```python
from build123d import *

# Parameters (mm, degrees)
SKIZZE1_W                       = 10
SKIZZE1_H                       = 11
AUFSATZ_LINEAR_AUSTRAGEN1_DEPTH = 9
SKIZZE2_W                       = 1.5
SKIZZE2_H                       = 1
AUFSATZ_LINEAR_AUSTRAGEN2_DEPTH = 9
SKIZZE6_W                       = 3.75
SKIZZE6_H                       = 3.75
SCHNITT_LINEAR_AUSTRAGEN2_DEPTH = 10
LINEARES_MUSTER1_COUNT          = 4
LINEARES_MUSTER1_PITCH          = 4.25
LINEARES_MUSTER1_COUNT_DIR2     = 2
LINEARES_MUSTER1_PITCH_DIR2     = 4.25
SKIZZE7_W                       = 3.5
SKIZZE7_H                       = 3.5
AUFSATZ_LINEAR_AUSTRAGEN5_DEPTH = 9
LINEARES_MUSTER2_COUNT          = 3
LINEARES_MUSTER2_PITCH          = 4.25
LINEARES_MUSTER2_COUNT_DIR2     = 2
LINEARES_MUSTER2_PITCH_DIR2     = 4.25
AUFSATZ_LINEAR_AUSTRAGEN7_DEPTH = 9
LINEARES_MUSTER4_COUNT          = 4
LINEARES_MUSTER4_PITCH          = 4.25
LINEARES_MUSTER4_COUNT_DIR2     = 2
LINEARES_MUSTER4_PITCH_DIR2     = 4.25
SCHNITT_LINEAR_AUSTRAGEN4_DEPTH = 23.874658467
LINEARES_MUSTER6_COUNT          = 4
LINEARES_MUSTER6_PITCH          = 4.25
LINEARES_MUSTER6_COUNT_DIR2     = 2
LINEARES_MUSTER6_PITCH_DIR2     = 4.25
SKETCH_3_W                      = 20.071123044
SKETCH_3_H                      = 21.030403289
CUT_EXTRUDE_1_DEPTH             = 8


with BuildPart() as part:
    # Skizze1 → Aufsatz-Linear austragen1 (new, symmetric)
    with BuildSketch(Plane(origin=(0, 0, 0), x_dir=(0, 0, -1), z_dir=(1, 0, 0))):
        with Locations((0, 5.5)):
            Rectangle(SKIZZE1_W, SKIZZE1_H)
    extrude(amount=AUFSATZ_LINEAR_AUSTRAGEN1_DEPTH, both=True)

    # Skizze2 → Aufsatz-Linear austragen2 (add, symmetric)
    with BuildSketch(Plane(origin=(0, 0, 0), x_dir=(0, 0, -1), z_dir=(1, 0, 0))):
        with Locations((-5.75, 0.5)):
            Rectangle(SKIZZE2_W, SKIZZE2_H)
        with Locations((5.75, 0.5)):
            Rectangle(SKIZZE2_W, SKIZZE2_H)
    extrude(amount=AUFSATZ_LINEAR_AUSTRAGEN2_DEPTH, both=True)

    # Skizze6 → Schnitt-Linear austragen2 (cut)
    with BuildSketch(Plane.XZ):
        with Locations((-6.375, -2.125)):
            Rectangle(SKIZZE6_W, SKIZZE6_H)
    schnitt_linear_austragen2 = extrude(amount=-SCHNITT_LINEAR_AUSTRAGEN2_DEPTH, mode=Mode.SUBTRACT)

    # Lineares Muster1: Schnitt-Linear austragen2 4 × 2
    with Locations(*[(i * LINEARES_MUSTER1_PITCH, 0, j * LINEARES_MUSTER1_PITCH_DIR2) for i in range(LINEARES_MUSTER1_COUNT) for j in range(LINEARES_MUSTER1_COUNT_DIR2) if (i, j) != (0, 0)]):
        add(schnitt_linear_austragen2, mode=Mode.SUBTRACT)

    # Skizze7 → Aufsatz-Linear austragen5 (add)
    with BuildSketch(Plane(origin=(0, 11, 0), x_dir=(1, 0, 0), z_dir=(0, 1, 0))):
        with Locations((-6.375, -2.125)):
            Rectangle(SKIZZE7_W, SKIZZE7_H)
    aufsatz_linear_austragen5 = extrude(amount=AUFSATZ_LINEAR_AUSTRAGEN5_DEPTH)

    # Lineares Muster2: Aufsatz-Linear austragen5 3 × 2, 4 skipped
    with Locations(*[(i * LINEARES_MUSTER2_PITCH, 0, -j * LINEARES_MUSTER2_PITCH_DIR2) for i in range(LINEARES_MUSTER2_COUNT) for j in range(LINEARES_MUSTER2_COUNT_DIR2) if (i, j) not in ((0, 0), (0, 1), (1, 0), (1, 1), (2, 0))]):
        add(aufsatz_linear_austragen5)

    # Skizze10 → Aufsatz-Linear austragen7 (add)
    with BuildSketch(Plane(origin=(0, 11, 0), x_dir=(1, 0, 0), z_dir=(0, 1, 0))):
        Polygon((-4.625, 1.375), (-5.625, 0.375), (-7.125, 0.375), (-8.125, 1.375), (-8.125, 3.875), (-4.625, 3.875), align=None)
    aufsatz_linear_austragen7 = extrude(amount=AUFSATZ_LINEAR_AUSTRAGEN7_DEPTH)

    # Lineares Muster4: Aufsatz-Linear austragen7 4 × 2, 2 skipped
    with Locations(*[(i * LINEARES_MUSTER4_PITCH, 0, j * LINEARES_MUSTER4_PITCH_DIR2) for i in range(LINEARES_MUSTER4_COUNT) for j in range(LINEARES_MUSTER4_COUNT_DIR2) if (i, j) not in ((0, 0), (0, 1), (2, 0))]):
        add(aufsatz_linear_austragen7)

    # Skizze12 → Schnitt-Linear austragen4 (cut, through all)
    with BuildSketch(Plane(origin=(0, 20, 0), x_dir=(1, 0, 0), z_dir=(0, 1, 0))):
        Polygon((-5.875, 0.875), (-5.125, 1.625), (-5.125, 3.375), (-7.625, 3.375), (-7.625, 1.625), (-6.875, 0.875), align=None)
    schnitt_linear_austragen4 = extrude(amount=-SCHNITT_LINEAR_AUSTRAGEN4_DEPTH, mode=Mode.SUBTRACT)

    # Lineares Muster6: Schnitt-Linear austragen4 4 × 2
    with Locations(*[(i * LINEARES_MUSTER6_PITCH, 0, j * LINEARES_MUSTER6_PITCH_DIR2) for i in range(LINEARES_MUSTER6_COUNT) for j in range(LINEARES_MUSTER6_COUNT_DIR2) if (i, j) != (0, 0)]):
        add(schnitt_linear_austragen4, mode=Mode.SUBTRACT)

    # 草图3 → 切除-拉伸1 (cut)
    with BuildSketch(Plane(origin=(0, 0, 0), x_dir=(-1, 0, 0), z_dir=(0, -1, 0))):
        with Locations((-0.428033297, -0.424589463)):
            Rectangle(SKETCH_3_W, SKETCH_3_H)
    extrude(amount=-CUT_EXTRUDE_1_DEPTH, mode=Mode.SUBTRACT)


solid = part.part
```
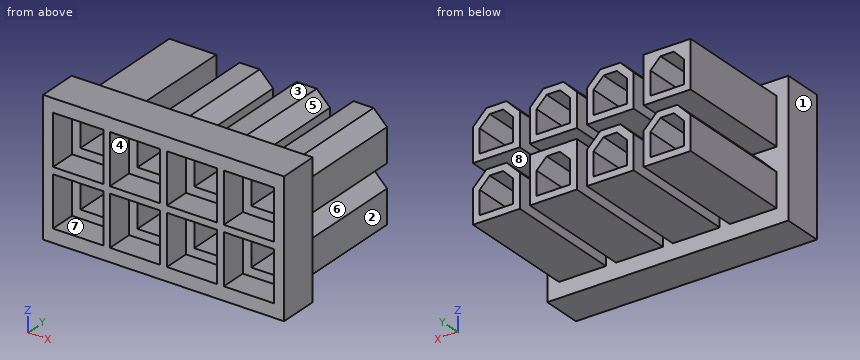
Verification items for the finished model (mm, model axes). Face numbers are marked on the shaded views. A direction names the side the tool comes from. Coordinates: 2 decimals unless noted, no trailing zeros. Loops run counter-clockwise (first coordinate to the right, second up) from the corner with the lowest first, then second, coordinate; pieces in that order, holes last. Notation, with made-up numbers: (11.5, 60.5) - (51.5, 60.5) arc R23 cw to (51.5, 77.5) - close; hole circle Ø3 at (65.25, 68.25). An arc over 180 degrees is marked (long way). Answer as a JSON object with one key per item and string values.
(1) Mould release check, pull along X, two halves, no side actions. Record for the marked faces 1, 2, 3 and 4: pulls with the +X half, pulls with the -X half, needs draft (parallel to the pull), parting line crosses it, or undercut.
Response:
{"face 1": "pulls with the -X half", "face 2": "pulls with the +X half", "face 3": "needs draft", "face 4": "undercut"}
(2) Scan lines: line 1 along Z through (x, y) = (2.5, 15.5) (3 decimals); line 2 along X through (y, z) = (13.5, -3.75) (3 decimals); line 3 along Z through (x, y) = (-2, 9). Record each from-to range of solid material in increasing order.
Response:
{"line 1": "z = -3.875 to -3.375, -0.875 to -0.375, 0.375 to 0.875, 3.375 to 3.875", "line 2": "x = -8.125 to -4.625, -3.875 to -0.375, 0.375 to 3.875, 4.625 to 8.125", "line 3": "z = -5 to -4, -0.25 to 0.25, 4 to 5"}
(3) Go/stop test with flat-tipped pins: pin 1 Ø1.4 at (y, z) = (16.5, -2) entering from -X (3 decimals); pin 2 Ø0.8 at (x, y) = (2.5, 17) entering from +Z (3 decimals); pin 3 Ø0.9 at (y, z) = (14.5, 1.5) entering from +X (3 decimals). Record where each tip stops, or that it passes through.
Response:
{"pin 1": "stops at x = -8.125", "pin 2": "stops at z = 3.875", "pin 3": "stops at x = 8.125"}
(4) Cross-section at D-D, the plane z = 0. Record the boundary of the cut face in (x, y), then the cut area to 3 significant figures.
Response:
{"outline": "(-9, 8) - (9, 8) - (9, 11) - (-9, 11) - close", "area": "54.0 mm²"}
(5) Cross-section at A-A, the plane x = 2.25. Record the boundary of the cut face in (y, z) (3 decimals).
Response:
{"outline": "(8, -5) - (11, -5) - (11, -3.875) - (20, -3.875) - (20, -3.375) - (10, -3.375) - (10, -4) - (8, -4) - close; (8, -0.25) - (10, -0.25) - (10, -0.875) - (20, -0.875) - (20, -0.375) - (11, -0.375) - (11, 0.375) - (20, 0.375) - (20, 0.875) - (10, 0.875) - (10, 0.25) - (8, 0.25) - close; (8, 4) - (10, 4) - (10, 3.375) - (20, 3.375) - (20, 3.875) - (11, 3.875) - (11, 5) - (8, 5) - close"}
(6) Access from +Z, -Z, +X, -X, +Y, -Y to the whole of each face (thin tool, end or side, straight path). Record for the marked faces 5, 6, 7 and 8.
Response:
{"face 5": "+Z, +Y", "face 6": "+X, +Y", "face 7": "-Y", "face 8": "+X, -X, +Y"}
(7) Cross-section at B-B, the plane y = 16. Count the separate pieces of the cut face and the enclosed holes in it, then the cut area to 3 significant figures.
Response:
{"separate pieces": "8", "enclosed holes": "8", "area": "46.5 mm²"}
